Verification items for the finished model (mm, model axes). Round coordinates to 2 decimals unless told otherwise and drop trailing zeros. Write each loop counter-clockwise with the first axis right and the second up, starting at its lowest first coordinate (ties: lowest second). Pieces come first, ordered by that corner, then holes. Notation, with made-up numbers: (-14, 55.25) - (-3, 55.25) arc R16 ccw to (-3, 66.25) - close; hole circle Ø10 at (42, 0). An arc over 180 degrees is marked (long way). Answer as a JSON object with one key per item and string values. Group by question number.
1) Thickness scan on line 1 (X direction, y = 0.3, z = 5.75); line 2 (Z direction, x = 3, y = 0.1); line 3 (Z direction, x = -1.5, y = 0.5). Record the ranges inside material, lowest first.
2) Go/stop test with a flat-tipped pin: pin 1 Ø5 at (x, z) = (2, -1) entering from -Y. Record where the tip stops, or that it passes through.
3) Section check A-A (z = 0). Enter the section's corners in (x, y).
4) Section check B-B (x = 0). Enter the section's corners in (y, z).
```python
from build123d import *

# Parameters (mm, degrees)
SKETCH1_R           = 7.94
SKETCH1_R_2         = 6.5
BOSS_EXTRUDE1_DEPTH = 0.57
CUT_EXTRUDE1_DEPTH  = 1.57


with BuildPart() as part:
    # Sketch1 → Boss-Extrude1 (new body)
    with BuildSketch(Plane(origin=(0, 0, 0), x_dir=(1, 0, 0), z_dir=(0, 1, 0))):
        Circle(SKETCH1_R)
        Circle(SKETCH1_R_2, mode=Mode.SUBTRACT)
    extrude(amount=BOSS_EXTRUDE1_DEPTH)

    # Sketch2 → Cut-Extrude1 (cut, through all)
    with BuildSketch(Plane(origin=(0, 0.57, 0), x_dir=(1, 0, 0), z_dir=(0, 1, 0))):
        with BuildLine():
            Line((-0.35, 7.031294333), (-0.323153409, 6.491962097))
            ThreePointArc((-0.323153409, 6.491962097), (0, 6.5), (0.323153409, 6.491962097))
            Line((0.323153409, 6.491962097), (0.35, 7.031294333))
            ThreePointArc((0.35, 7.031294333), (0, 7.04), (-0.35, 7.031294333))
        make_face()
        with BuildLine():
            Line((1.804239954, 6.80487459), (1.665846548, 6.282909778))
            ThreePointArc((1.665846548, 6.282909778), (1.35142599, 6.357959405), (1.033663085, 6.417284521))
            Line((1.033663085, 6.417284521), (1.119536633, 6.950412774))
            ThreePointArc((1.119536633, 6.950412774), (1.463698303, 6.886159109), (1.804239954, 6.80487459))
        make_face()
        with BuildLine():
            Line((3.179625964, 6.281049174), (2.935734199, 5.799264152))
            ThreePointArc((2.935734199, 5.799264152), (2.64378818, 5.938045475), (2.345303541, 6.062140818))
            Line((2.345303541, 6.062140818), (2.540144143, 6.565764825))
            ThreePointArc((2.540144143, 6.565764825), (2.863425967, 6.431360022), (3.179625964, 6.281049174))
        make_face()
        with BuildLine():
            Line((4.416047062, 5.48271177), (4.077316179, 5.062162856))
            ThreePointArc((4.077316179, 5.062162856), (3.82060414, 5.258610463), (3.55444298, 5.442052472))
            Line((3.55444298, 5.442052472), (3.849735166, 5.894161446))
            ThreePointArc((3.849735166, 5.894161446), (4.138008176, 5.69547964), (4.416047062, 5.48271177))
        make_face()
        with BuildLine():
            Line((5.459465712, 4.444753552), (5.040699876, 4.103820751))
            ThreePointArc((5.040699876, 4.103820751), (4.830441366, 4.349348941), (4.608236203, 4.584120318))
            Line((4.608236203, 4.584120318), (4.991074288, 4.96495493))
            ThreePointArc((4.991074288, 4.96495493), (5.231739571, 4.710679469), (5.459465712, 4.444753552))
        make_face()
        with BuildLine():
            Line((6.264279514, 3.212538275), (5.783780801, 2.966121987))
            ThreePointArc((5.783780801, 2.966121987), (5.629165125, 3.25), (5.460627392, 3.52584011))
            Line((5.460627392, 3.52584011), (5.914279514, 3.818756058))
            ThreePointArc((5.914279514, 3.818756058), (6.096818843, 3.52), (6.264279514, 3.212538275))
        make_face()
        with BuildLine():
            Line((6.795314242, 1.839919661), (6.274082751, 1.698789459))
            ThreePointArc((6.274082751, 1.698789459), (6.181867356, 2.008610463), (6.074362961, 2.31346377))
            Line((6.074362961, 2.31346377), (6.579002346, 2.505659222))
            ThreePointArc((6.579002346, 2.505659222), (6.695437875, 2.17547964), (6.795314242, 1.839919661))
        make_face()
        with BuildLine():
            Line((7.029361129, 0.386887728), (6.490177179, 0.357211681))
            ThreePointArc((6.490177179, 0.357211681), (6.46439232, 0.679435011), (6.422619721, 0.999977963))
            Line((6.422619721, 0.999977963), (6.956191205, 1.083053055))
            ThreePointArc((6.956191205, 1.083053055), (7.001434143, 0.735880381), (7.029361129, 0.386887728))
        make_face()
        with BuildLine():
            Line((6.956191205, -1.083053055), (6.422619721, -0.999977963))
            ThreePointArc((6.422619721, -0.999977963), (6.46439232, -0.679435011), (6.490177179, -0.357211681))
            Line((6.490177179, -0.357211681), (7.029361129, -0.386887728))
            ThreePointArc((7.029361129, -0.386887728), (7.001434143, -0.735880381), (6.956191205, -1.083053055))
        make_face()
        with BuildLine():
            Line((6.579002346, -2.505659222), (6.074362961, -2.31346377))
            ThreePointArc((6.074362961, -2.31346377), (6.181867356, -2.008610463), (6.274082751, -1.698789459))
            Line((6.274082751, -1.698789459), (6.795314242, -1.839919661))
            ThreePointArc((6.795314242, -1.839919661), (6.695437875, -2.17547964), (6.579002346, -2.505659222))
        make_face()
        with BuildLine():
            Line((5.914279514, -3.818756058), (5.460627392, -3.52584011))
            ThreePointArc((5.460627392, -3.52584011), (5.629165125, -3.25), (5.783780801, -2.966121987))
            Line((5.783780801, -2.966121987), (6.264279514, -3.212538275))
            ThreePointArc((6.264279514, -3.212538275), (6.096818843, -3.52), (5.914279514, -3.818756058))
        make_face()
        with BuildLine():
            Line((4.991074288, -4.96495493), (4.608236203, -4.584120318))
            ThreePointArc((4.608236203, -4.584120318), (4.830441366, -4.349348941), (5.040699876, -4.103820751))
            Line((5.040699876, -4.103820751), (5.459465712, -4.444753552))
            ThreePointArc((5.459465712, -4.444753552), (5.231739571, -4.710679469), (4.991074288, -4.96495493))
        make_face()
        with BuildLine():
            Line((3.849735166, -5.894161446), (3.55444298, -5.442052472))
            ThreePointArc((3.55444298, -5.442052472), (3.82060414, -5.258610463), (4.077316179, -5.062162856))
            Line((4.077316179, -5.062162856), (4.416047062, -5.48271177))
            ThreePointArc((4.416047062, -5.48271177), (4.138008176, -5.69547964), (3.849735166, -5.894161446))
        make_face()
        with BuildLine():
            Line((2.540144143, -6.565764825), (2.345303541, -6.062140818))
            ThreePointArc((2.345303541, -6.062140818), (2.64378818, -5.938045475), (2.935734199, -5.799264152))
            Line((2.935734199, -5.799264152), (3.179625964, -6.281049174))
            ThreePointArc((3.179625964, -6.281049174), (2.863425967, -6.431360022), (2.540144143, -6.565764825))
        make_face()
        with BuildLine():
            Line((1.119536633, -6.950412774), (1.033663085, -6.417284521))
            ThreePointArc((1.033663085, -6.417284521), (1.35142599, -6.357959405), (1.665846548, -6.282909778))
            Line((1.665846548, -6.282909778), (1.804239954, -6.80487459))
            ThreePointArc((1.804239954, -6.80487459), (1.463698303, -6.886159109), (1.119536633, -6.950412774))
        make_face()
        with BuildLine():
            Line((-0.35, -7.031294333), (-0.323153409, -6.491962097))
            ThreePointArc((-0.323153409, -6.491962097), (0, -6.5), (0.323153409, -6.491962097))
            Line((0.323153409, -6.491962097), (0.35, -7.031294333))
            ThreePointArc((0.35, -7.031294333), (0, -7.04), (-0.35, -7.031294333))
        make_face()
        with BuildLine():
            Line((-1.804239954, -6.80487459), (-1.665846548, -6.282909778))
            ThreePointArc((-1.665846548, -6.282909778), (-1.35142599, -6.357959405), (-1.033663085, -6.417284521))
            Line((-1.033663085, -6.417284521), (-1.119536633, -6.950412774))
            ThreePointArc((-1.119536633, -6.950412774), (-1.463698303, -6.886159109), (-1.804239954, -6.80487459))
        make_face()
        with BuildLine():
            Line((-3.179625964, -6.281049174), (-2.935734199, -5.799264152))
            ThreePointArc((-2.935734199, -5.799264152), (-2.64378818, -5.938045475), (-2.345303541, -6.062140818))
            Line((-2.345303541, -6.062140818), (-2.540144143, -6.565764825))
            ThreePointArc((-2.540144143, -6.565764825), (-2.863425967, -6.431360022), (-3.179625964, -6.281049174))
        make_face()
        with BuildLine():
            Line((-4.416047062, -5.48271177), (-4.077316179, -5.062162856))
            ThreePointArc((-4.077316179, -5.062162856), (-3.82060414, -5.258610463), (-3.55444298, -5.442052472))
            Line((-3.55444298, -5.442052472), (-3.849735166, -5.894161446))
            ThreePointArc((-3.849735166, -5.894161446), (-4.138008176, -5.69547964), (-4.416047062, -5.48271177))
        make_face()
        with BuildLine():
            Line((-5.459465712, -4.444753552), (-5.040699876, -4.103820751))
            ThreePointArc((-5.040699876, -4.103820751), (-4.830441366, -4.349348941), (-4.608236203, -4.584120318))
            Line((-4.608236203, -4.584120318), (-4.991074288, -4.96495493))
            ThreePointArc((-4.991074288, -4.96495493), (-5.231739571, -4.710679469), (-5.459465712, -4.444753552))
        make_face()
        with BuildLine():
            Line((-6.264279514, -3.212538275), (-5.783780801, -2.966121987))
            ThreePointArc((-5.783780801, -2.966121987), (-5.629165125, -3.25), (-5.460627392, -3.52584011))
            Line((-5.460627392, -3.52584011), (-5.914279514, -3.818756058))
            ThreePointArc((-5.914279514, -3.818756058), (-6.096818843, -3.52), (-6.264279514, -3.212538275))
        make_face()
        with BuildLine():
            Line((-6.795314242, -1.839919661), (-6.274082751, -1.698789459))
            ThreePointArc((-6.274082751, -1.698789459), (-6.181867356, -2.008610463), (-6.074362961, -2.31346377))
            Line((-6.074362961, -2.31346377), (-6.579002346, -2.505659222))
            ThreePointArc((-6.579002346, -2.505659222), (-6.695437875, -2.17547964), (-6.795314242, -1.839919661))
        make_face()
        with BuildLine():
            Line((-7.029361129, -0.386887728), (-6.490177179, -0.357211681))
            ThreePointArc((-6.490177179, -0.357211681), (-6.46439232, -0.679435011), (-6.422619721, -0.999977963))
            Line((-6.422619721, -0.999977963), (-6.956191205, -1.083053055))
            ThreePointArc((-6.956191205, -1.083053055), (-7.001434143, -0.735880381), (-7.029361129, -0.386887728))
        make_face()
        with BuildLine():
            Line((-6.956191205, 1.083053055), (-6.422619721, 0.999977963))
            ThreePointArc((-6.422619721, 0.999977963), (-6.46439232, 0.679435011), (-6.490177179, 0.357211681))
            Line((-6.490177179, 0.357211681), (-7.029361129, 0.386887728))
            ThreePointArc((-7.029361129, 0.386887728), (-7.001434143, 0.735880381), (-6.956191205, 1.083053055))
        make_face()
        with BuildLine():
            Line((-6.579002346, 2.505659222), (-6.074362961, 2.31346377))
            ThreePointArc((-6.074362961, 2.31346377), (-6.181867356, 2.008610463), (-6.274082751, 1.698789459))
            Line((-6.274082751, 1.698789459), (-6.795314242, 1.839919661))
            ThreePointArc((-6.795314242, 1.839919661), (-6.695437875, 2.17547964), (-6.579002346, 2.505659222))
        make_face()
        with BuildLine():
            Line((-5.914279514, 3.818756058), (-5.460627392, 3.52584011))
            ThreePointArc((-5.460627392, 3.52584011), (-5.629165125, 3.25), (-5.783780801, 2.966121987))
            Line((-5.783780801, 2.966121987), (-6.264279514, 3.212538275))
            ThreePointArc((-6.264279514, 3.212538275), (-6.096818843, 3.52), (-5.914279514, 3.818756058))
        make_face()
        with BuildLine():
            Line((-4.991074288, 4.96495493), (-4.608236203, 4.584120318))
            ThreePointArc((-4.608236203, 4.584120318), (-4.830441366, 4.349348941), (-5.040699876, 4.103820751))
            Line((-5.040699876, 4.103820751), (-5.459465712, 4.444753552))
            ThreePointArc((-5.459465712, 4.444753552), (-5.231739571, 4.710679469), (-4.991074288, 4.96495493))
        make_face()
        with BuildLine():
            Line((-3.849735166, 5.894161446), (-3.55444298, 5.442052472))
            ThreePointArc((-3.55444298, 5.442052472), (-3.82060414, 5.258610463), (-4.077316179, 5.062162856))
            Line((-4.077316179, 5.062162856), (-4.416047062, 5.48271177))
            ThreePointArc((-4.416047062, 5.48271177), (-4.138008176, 5.69547964), (-3.849735166, 5.894161446))
        make_face()
        with BuildLine():
            Line((-2.540144143, 6.565764825), (-2.345303541, 6.062140818))
            ThreePointArc((-2.345303541, 6.062140818), (-2.64378818, 5.938045475), (-2.935734199, 5.799264152))
            Line((-2.935734199, 5.799264152), (-3.179625964, 6.281049174))
            ThreePointArc((-3.179625964, 6.281049174), (-2.863425967, 6.431360022), (-2.540144143, 6.565764825))
        make_face()
        with BuildLine():
            Line((-1.119536633, 6.950412774), (-1.033663085, 6.417284521))
            ThreePointArc((-1.033663085, 6.417284521), (-1.35142599, 6.357959405), (-1.665846548, 6.282909778))
            Line((-1.665846548, 6.282909778), (-1.804239954, 6.80487459))
            ThreePointArc((-1.804239954, 6.80487459), (-1.463698303, 6.886159109), (-1.119536633, 6.950412774))
        make_face()
    extrude(amount=-CUT_EXTRUDE1_DEPTH, mode=Mode.SUBTRACT)


solid = part.part
```
Returned:
{
 "1": {"line 1": "-5.48 to -4.06, -3.76 to -3.03, 3.03 to 3.76, 4.06 to 5.48", "line 2": "-7.35 to -6.37, -5.93 to -5.77, 5.77 to 5.93, 6.37 to 7.35", "line 3": "-7.8 to -6.88, 6.88 to 7.8"},
 "2": {"pin 1": "through"},
 "3": {"outline": "(-7.94, 0) - (-6.5, 0) - (-6.5, 0.57) - (-7.94, 0.57) - close; (6.5, 0) - (7.94, 0) - (7.94, 0.57) - (6.5, 0.57) - close"},
 "4": {"outline": "(0, -7.94) - (0.57, -7.94) - (0.57, -7.04) - (0, -7.04) - close; (0, 7.04) - (0.57, 7.04) - (0.57, 7.94) - (0, 7.94) - close"}
}
